from build123d import *

# Parameters (mm, degrees)
F0_R     = 29
F0_R_2   = 2
F0_R_3   = 2.1
F0_R_4   = 4
F1_DEPTH = 6


with BuildPart() as f1:
    # F0 (on Right) → F1 (new body)
    with BuildSketch(Plane.YZ):
        Circle(F0_R)
        with Locations((-7.5, -12.990381)):
            Circle(F0_R_2, mode=Mode.SUBTRACT)
        with Locations((-12.557368, -7.25)):
            Circle(F0_R_3, mode=Mode.SUBTRACT)
        with Locations((7.5, -12.990381)):
            Circle(F0_R_2, mode=Mode.SUBTRACT)
        with Locations((12.557368, -7.25)):
            Circle(F0_R_3, mode=Mode.SUBTRACT)
        with Locations((-15, 0)):
            Circle(F0_R_2, mode=Mode.SUBTRACT)
        with Locations((-7.5, 12.990381)):
            Circle(F0_R_2, mode=Mode.SUBTRACT)
        Circle(F0_R_4, mode=Mode.SUBTRACT)
        with Locations((7.5, 12.990381)):
            Circle(F0_R_2, mode=Mode.SUBTRACT)
        with Locations((15, 0)):
            Circle(F0_R_2, mode=Mode.SUBTRACT)
        with Locations((0, 14.5)):
            Circle(F0_R_3, mode=Mode.SUBTRACT)
    extrude(amount=F1_DEPTH)


solid = f1.part
Design review of the part built by this model. Coordinates are the model's own, in mm. Give positions to 0.01 mm unless a question says otherwise; leave off trailing zeros. Loops run counter-clockwise (first coordinate to the right, second up) from the corner with the lowest first, then second, coordinate; pieces in that order, holes last. Notation, with made-up numbers: M 72,47.25 L 85,47.25 A29 ccw 85,70.25 Z; hole C 55.5,59.5 d9. An arc over 180 degrees is marked long. Write item = value, one per line.
Q1. Draft analysis for pull direction Z (two halves, no side actions). For faces 1 (the cylindrical face through (2.958, 5.913, 11.773)), 2 (the flat face through (6, 6, 0)), 3 (the cylindrical face through (2.96, 13.38, -25.73)), state which applies: +Z half, -Z half, draft (parallel to the pull), parting line (faces both ways), or undercut.
Output values:
face_1 = undercut
face_2 = draft
face_3 = parting line
Q2. We need section C-C (x = 3.4). Count the separate pieces of the cut face and the enclosed holes in it, plus the area to 3 significant figures.
Output values:
separate_pieces = 1
enclosed_holes = 10
area = 2,470 mm^2
Q3. Insertion check: pin 1 (1.5 mm diameter, centred on x = 1, z = -22, fed in from -Y); pin 2 (1.5 mm diameter, centred on x = 5.5, y = 19, fed in from -Z). Each pin has a flat end and moves straight along its axis. Give the tip position at first contact, or say it passes through.
Output values:
pin_1 = -19.73
pin_2 = -22.54
Q4. We need section D-D (y = -7.5). Give the boundary of the cut face in (x, z), plus the area to 3 significant figures.
Output values:
outline = M 0,-28.01 L 6,-28.01 L 6,-14.99 L 0,-14.99 Z; M 0,-10.99 L 6,-10.99 L 6,10.99 L 0,10.99 Z; M 0,14.99 L 6,14.99 L 6,28.01 L 0,28.01 Z
area = 288 mm^2
Q5. We need section B-B (y = 0). Give the boundary of the cut face in (x, z).
Output values:
outline = M 0,-29 L 6,-29 L 6,-4 L 0,-4 Z; M 0,4 L 6,4 L 6,12.4 L 0,12.4 Z; M 0,16.6 L 6,16.6 L 6,29 L 0,29 Z
Q6. We need section A-A (z = 0). Give the boundary of the cut face in (x, y).
Output values:
outline = M 0,-29 L 6,-29 L 6,-17 L 0,-17 Z; M 0,-13 L 6,-13 L 6,-4 L 0,-4 Z; M 0,4 L 6,4 L 6,13 L 0,13 Z; M 0,17 L 6,17 L 6,29 L 0,29 Z
Q7. To check wall thickness, follow line 1 (Z direction, x = 4.7, y = 0); line 2 (Z direction, x = 2.65, y = 7.5); line 3 (Z direction, x = 3.05, y = 12.5). State the ranges of each line that lie inside material, in increasing order. Write a range as [from, to].
Output values:
line_1 = [-29, -4], [4, 12.4], [16.6, 29]
line_2 = [-28.01, -14.99], [-10.99, 10.99], [14.99, 28.01]
line_3 = [-26.17, -9.35], [-5.15, 26.17]
